from build123d import *

# Parameters (mm, degrees)
BOSS_EXTRUDE1_DEPTH = 30
SKETCH2_R           = 1.5
CUT_EXTRUDE1_DEPTH  = 53
SKETCH3_R           = 6.25
SKETCH3_R_2         = 1.5
CUT_EXTRUDE2_DEPTH  = 30
FILLET1_R           = 2


with BuildPart() as part:
    # Sketch1 → Boss-Extrude1 (new body)
    with BuildSketch(Plane(origin=(0, 0, 0), x_dir=(1, 0, 0), z_dir=(0, 1, 0))):
        Polygon((24, 0), (24, -25), (-24, -25), (-24, 0), (-26, 0), (-26, -27), (26, -27), (26, 0), align=None)
    extrude(amount=BOSS_EXTRUDE1_DEPTH)

    # Sketch2 → Cut-Extrude1 (cut, through all)
    with BuildSketch(Plane(origin=(26, 0, 0), x_dir=(0, 0, -1), z_dir=(1, 0, 0))):
        with Locations((-4, 27)):
            Circle(SKETCH2_R)
        with Locations((-4, 3)):
            Circle(SKETCH2_R)
        with Locations((-16, 15)):
            Circle(SKETCH2_R)
        with Locations((-16, 27)):
            Circle(SKETCH2_R)
        with Locations((-16, 3)):
            Circle(SKETCH2_R)
        with BuildLine():
            Line((-4.25, 21.25), (0, 21.25))
            Line((0, 21.25), (0, 8.75))
            Line((0, 8.75), (-4.25, 8.75))
            ThreePointArc((-4.25, 8.75), (-10.5, 15), (-4.25, 21.25))
        make_face()
    extrude(amount=-CUT_EXTRUDE1_DEPTH, mode=Mode.SUBTRACT)

    # Sketch3 → Cut-Extrude2 (cut)
    with BuildSketch(Plane.XY.offset(27)):
        with Locations((0, 15)):
            Circle(SKETCH3_R)
        with Locations((20, 23.5)):
            Circle(SKETCH3_R_2)
        with Locations((20, 6.5)):
            Circle(SKETCH3_R_2)
        with Locations((8.5, 6.5)):
            Circle(SKETCH3_R_2)
        with Locations((8.5, 23.5)):
            Circle(SKETCH3_R_2)
        with Locations((-8.5, 6.5)):
            Circle(SKETCH3_R_2)
        with Locations((-20, 6.5)):
            Circle(SKETCH3_R_2)
        with Locations((-8.5, 23.5)):
            Circle(SKETCH3_R_2)
        with Locations((-20, 23.5)):
            Circle(SKETCH3_R_2)
    extrude(amount=-CUT_EXTRUDE2_DEPTH, mode=Mode.SUBTRACT)

    # Fillet1
    fillet1_edges = [part.edges().sort_by_distance(p)[0] for p in [
        (25, 0, 0),
        (26, 15, 27),
        (-26, 15, 27),
        (-25, 30, 0),
        (25, 30, 0),
        (25, 21.25, 0),
        (-25, 21.25, 0),
        (25, 8.75, 0),
        (-25, 8.75, 0),
        (-25, 0, 0),
    ]]
    fillet(fillet1_edges, radius=FILLET1_R)


solid = part.part
The listing builds one solid part. Answer for the finished solid, in the listing's coordinates (mm). A direction names the side the tool comes from. Round coordinates to 2 decimals unless told otherwise and drop trailing zeros. Order: outer loops, then holes, each group sorted by start corner. A loop starts at its lowest first (then second) coordinate and runs counter-clockwise, first axis right, second up. Notation, with made-up numbers: M 10,-35.75 L 33,-35.75 A35 cw 33,-2.75 Z; hole C -24.5,5 d4. An arc over 180 degrees is marked long. Answer in a Markdown table with one row per item. Add a question column.
1) The part is cut by section D-D on y = 27. Determine the outline of the cut face in (x, z).
2) Which of the six approach directions +Z, -Z, +X, -X, +Y, -Y give full straight-line access (tool end or side, diameter ignored) to faces 4 (the face through (26, 15, 13)), 5 (the face through (-25.01, 8.15, 0.57)), 6 (the face through (-24, 15, 13))?
3) A flat-ended cylindrical pin translates along its axis: pin 1 Ø10 at (x, y) = (-10, 26) entering from -Z. Find the tip coordinate at first contact, or state that the pin passes through.
4) The part is cut by section B-B on z = 19.5. Determine the outline of the cut face in (x, y).
5) The part is cut by section C-C on x = -8.5. Determine the outline of the cut face in (y, z).
6) The part is cut by section A-A on y = 15. Determine the outline of the cut face in (x, z).
7) Determine the mould class of faces 1 (the face through (-25, 14.9, 10.5)), 2 (the face through (-25, 26, 0)), 3 (the face through (24.99, 29.43, 0.6)) for opening direction Y: pulls with the +Y half, pulls with the -Y half, needs draft (parallel to the pull), parting line crosses it, or undercut.
8) Consider line 1 along Y through (x, z) = (25, 16); line 2 along Y through (x, z) = (24.5, 4); line 3 along Y through (x, z) = (-20, 25.95). Determine where each line is inside the solid, lowest interval first. Write a range as from..to.
Findings below:
| question | item | result |
|---|---|---|
| 1 | outline | M -26,0 L -24,0 L -24,2.5 L -26,2.5 Z; M -26,5.5 L -24,5.5 L -24,14.5 L -26,14.5 Z; M -26,17.5 L -24,17.5 L -24,25 L 24,25 L 24,17.5 L 26,17.5 L 26,25 A2 ccw 24,27 L -24,27 A2 ccw -26,25 Z; M 24,0 L 26,0 L 26,2.5 L 24,2.5 Z; M 24,5.5 L 26,5.5 L 26,14.5 L 24,14.5 Z |
| 2 | face 4 | +Z, -Z, +X, +Y, -Y |
| 2 | face 5 | -Z, +X, -X |
| 2 | face 6 | -Z, +Y, -Y |
| 3 | pin 1 | stops at z = 25 |
| 4 | outline | M -26,0 L -24,0 L -24,30 L -26,30 Z; M 24,0 L 26,0 L 26,30 L 24,30 Z |
| 5 | outline | M 0,25 L 5,25 L 5,27 L 0,27 Z; M 8,25 L 22,25 L 22,27 L 8,27 Z; M 25,25 L 30,25 L 30,27 L 25,27 Z |
| 6 | outline | M -26,10.5 L -24,10.5 L -24,14.5 L -26,14.5 Z; M -26,17.5 L -24,17.5 L -24,25 L -6.25,25 L -6.25,27 L -24,27 A2 ccw -26,25 Z; M 6.25,25 L 24,25 L 24,17.5 L 26,17.5 L 26,25 A2 ccw 24,27 L 6.25,27 Z; M 24,10.5 L 26,10.5 L 26,14.5 L 24,14.5 Z |
| 7 | face 1 | undercut |
| 7 | face 2 | needs draft |
| 7 | face 3 | pulls with the +Y half |
| 8 | line 1 | y = 0..1.5, 4.5..13.5, 16.5..25.5, 28.5..30 |
| 8 | line 2 | y = 0..1.5, 4.5..8.75, 21.25..25.5, 28.5..30 |
| 8 | line 3 | y = 0..5, 8..22, 25..30 |
